from build123d import *

# Parameters (mm, degrees)
SKETCH1_W           = 27
SKETCH1_H           = 50
SKETCH1_R           = 3
SKETCH1_R_2         = 1.75
BOSS_EXTRUDE1_DEPTH = 2
BOSS_EXTRUDE2_DEPTH = 12
SKETCH4_W           = 12
SKETCH4_H           = 7
CUT_EXTRUDE1_DEPTH  = 56.823382198


with BuildPart() as part:
    # Sketch1 → Boss-Extrude1 (new body)
    # profile 1 of 5: a face of its own
    with BuildSketch(Plane(origin=(0, 0, 0), x_dir=(1, 0, 0), z_dir=(0, 1, 0))):
        Rectangle(SKETCH1_W, SKETCH1_H)
    # profile 2 of 5: a face of its own
    with BuildSketch(Plane(origin=(0, 0, 0), x_dir=(1, 0, 0), z_dir=(0, 1, 0))):
        with BuildLine():
            Line((-17.5, -3), (-13.5, -3))
            Line((-13.5, -3), (-13.5, 3))
            Line((-13.5, 3), (-17.5, 3))
            ThreePointArc((-17.5, 3), (-15.378679656, 2.121320344), (-14.5, 0))
            ThreePointArc((-14.5, 0), (-15.378679656, -2.121320344), (-17.5, -3))
        make_face()
    # profile 3 of 5: a face of its own
    with BuildSketch(Plane(origin=(0, 0, 0), x_dir=(1, 0, 0), z_dir=(0, 1, 0))):
        with Locations((-17.5, 0)):
            Circle(SKETCH1_R)
        with Locations(Location((-17.5, 0, 0), (0, 0, 270))):
            Circle(SKETCH1_R_2, mode=Mode.SUBTRACT)
    # profile 4 of 5: a face of its own
    with BuildSketch(Plane(origin=(0, 0, 0), x_dir=(1, 0, 0), z_dir=(0, 1, 0))):
        with BuildLine():
            Line((13.5, 3), (13.5, -3))
            Line((13.5, -3), (17.5, -3))
            ThreePointArc((17.5, -3), (14.5, 0), (17.5, 3))
            Line((17.5, 3), (13.5, 3))
        make_face()
    # profile 5 of 5: a face of its own
    with BuildSketch(Plane(origin=(0, 0, 0), x_dir=(1, 0, 0), z_dir=(0, 1, 0))):
        with Locations((17.5, 0)):
            Circle(SKETCH1_R)
        with Locations(Location((17.5, 0, 0), (0, 0, 270))):
            Circle(SKETCH1_R_2, mode=Mode.SUBTRACT)
    extrude(amount=BOSS_EXTRUDE1_DEPTH)

    # Sketch2 → Boss-Extrude2 (add)
    with BuildSketch(Plane(origin=(0, 2, 0), x_dir=(1, 0, 0), z_dir=(0, 1, 0))):
        Polygon((-13.5, 25), (-13.5, -25), (13.5, -25), (13.5, 25), (12.5, 25), (12.5, -24), (-12.5, -24), (-12.5, 25), align=None)
    extrude(amount=BOSS_EXTRUDE2_DEPTH)

    # Sketch4 → Cut-Extrude1 (cut, through all)
    with BuildSketch(Plane.XY.offset(25)):
        with Locations((0, 5.5)):
            Rectangle(SKETCH4_W, SKETCH4_H)
    extrude(amount=-CUT_EXTRUDE1_DEPTH, mode=Mode.SUBTRACT)


solid = part.part
The model under review builds one solid part; all positions refer to its coordinate system, in mm. A direction names the side the tool comes from. Coordinates: 2 decimals unless noted, no trailing zeros. Loops run counter-clockwise (first coordinate to the right, second up) from the corner with the lowest first, then second, coordinate; pieces in that order, holes last. Notation, with made-up numbers: (0.5, 32.25) -> (38.5, 32.25) arc R12 cw to (38.5, 54.25) -> close; hole circle Ø4 at (17, 56.5). An arc over 180 degrees is marked (long way). Use a Markdown table: item, result. Add a question column.
1. Add section A-A on z = 0. Write out the cut boundary in (x, y), plus the area to 3 significant figures.
2. Draft analysis for pull direction Z (two halves, no side actions). For faces 1 (the face through (-16, 1, 3)), 2 (the face through (19.235, 0.986, -0.228)), 3 (the face through (-6, 5.5, 24.5)), state which applies: pulls with the +Z half, pulls with the -Z half, needs draft (parallel to the pull), parting line crosses it, or undercut.
3. Add section B-B on x = 5. Write out the cut boundary in (y, z).
4. Machinability: for faces 4 (the face through (12.5, 8, -1)), 5 (the face through (16, 1, -3)), 6 (the face through (-15, 1, -3)), 7 (the face through (-0.1, 9, 24.5)), which of the approach directions +Z, -Z, +X, -X, +Y, -Y give a long, thin tool a straight path to every point of the face, cutting with its end or side? Answer none if there is none.
5. Clearance check with flat-ended pins moving along their axes: pin 1 Ø0.5 at (y, z) = (4.5, 24.5) entering from +X; pin 2 Ø1 at (x, y) = (-15.5, 1.5) entering from +Z; pin 3 Ø4 at (x, z) = (-8, 19.5) entering from +Y. State where each tip first meets the part, or that it passes through.
6. To check wall thickness, follow line 1 (X direction, y = 0.7, z = 0); line 2 (X direction, y = 6.25, z = -18); line 3 (Y direction, x = 9, z = -10.5). State the ranges of each line that lie inside material, in increasing order.
7. Add section C-C on x = -9. Write out the cut boundary in (y, z).
Returned:
| question | item | result |
|---|---|---|
| 1 | outline | (-20.5, 0) -> (-19.25, 0) -> (-19.25, 2) -> (-20.5, 2) -> close; (-15.75, 0) -> (15.75, 0) -> (15.75, 2) -> (13.5, 2) -> (13.5, 14) -> (12.5, 14) -> (12.5, 2) -> (-12.5, 2) -> (-12.5, 14) -> (-13.5, 14) -> (-13.5, 2) -> (-15.75, 2) -> close; (19.25, 0) -> (20.5, 0) -> (20.5, 2) -> (19.25, 2) -> close |
| 1 | area | 92.0 mm² |
| 2 | face 1 | pulls with the +Z half |
| 2 | face 2 | undercut |
| 2 | face 3 | needs draft |
| 3 | outline | (0, -25) -> (2, -25) -> (2, 25) -> (0, 25) -> close; (9, 24) -> (14, 24) -> (14, 25) -> (9, 25) -> close |
| 4 | face 4 | -Z, +Y |
| 4 | face 5 | -Z, +X, +Y, -Y |
| 4 | face 6 | -Z, -X, +Y, -Y |
| 4 | face 7 | +Z, -Z |
| 5 | pin 1 | stops at x = 13.5 |
| 5 | pin 2 | stops at z = 3 |
| 5 | pin 3 | stops at y = 2 |
| 6 | line 1 | x = -20.5 to -19.25, -15.75 to 15.75, 19.25 to 20.5 |
| 6 | line 2 | x = -13.5 to -12.5, 12.5 to 13.5 |
| 6 | line 3 | y = 0 to 2 |
| 7 | outline | (0, -25) -> (2, -25) -> (2, 24) -> (14, 24) -> (14, 25) -> (0, 25) -> close |
